Read the model definition and answer for the solid it produces. Units are mm, in the model's axes. Coordinates: 2 decimals unless noted, no trailing zeros. Order: outer loops, then holes, each group sorted by start corner. A loop starts at its lowest first (then second) coordinate and runs counter-clockwise, first axis right, second up. Notation, with made-up numbers: (-15.75, 29) -> (14.25, 29) arc R28 ccw to (14.25, 51) -> close; hole circle Ø1 at (26, -20.75). An arc over 180 degrees is marked (long way). Use CSV: the item, a comma, the result in double quotes.
```python
from build123d import *

# Parameters (mm, degrees)
BOSS_EXTRUDE1_DEPTH = 1.6
CUT_EXTRUDE2_REACH  = 117.785
SKETCH2_4_W         = 3.3
SKETCH2_4_H         = 10


with BuildPart() as part:
    # Sketch1 → Boss-Extrude1 (new, symmetric)
    with BuildSketch(Plane.XY):
        with BuildLine():
            Line((-110, 0), (110, 0))
            ThreePointArc((110, 0), (113.989001648, -3.703578255), (110.591213415, -7.956067075))
            Line((110.591213415, -7.956067075), (30, -20))
            Line((30, -20), (0, -20))
            Line((0, -20), (-30, -20))
            Line((-30, -20), (-110.591213415, -7.956067075))
            ThreePointArc((-110.591213415, -7.956067075), (-113.989001648, -3.703578255), (-110, 0))
        make_face()
    extrude(amount=BOSS_EXTRUDE1_DEPTH, both=True)

    # Sketch2<4> → Cut-Extrude2 (cut, up to next)
    with BuildSketch(Plane.XY.offset(1.6), mode=Mode.PRIVATE) as cut_extrude2_sk1:
        with Locations((0, -5)):
            Rectangle(SKETCH2_4_W, SKETCH2_4_H)
    cut_extrude2_tool1 = extrude(cut_extrude2_sk1.sketch, amount=-CUT_EXTRUDE2_REACH, mode=Mode.PRIVATE) & part.part
    add(cut_extrude2_tool1.solids().sort_by_distance((0, -5, 1.6))[0], mode=Mode.SUBTRACT)


solid = part.part
```
Item 1: Find section D-D, the plane y = -14. Give the vertices of the cut face in (x, z), then the cut area to 3 significant figures.
Return value:
outline,"(-70.15, -1.6) -> (70.15, -1.6) -> (70.15, 1.6) -> (-70.15, 1.6) -> close"
area,"449 mm^2"
Item 2: Straight lines are drawn through the part: line 1 along X through (y, z) = (-4, -1.2); line 2 along X through (y, z) = (-4.75, 1.45); line 3 along Y through (x, z) = (73, -0.35). For each, find the intervals that lie inside material, in ascending order.
Return value:
line 1,"x = -114 to -1.65, 1.65 to 114"
line 2,"x = -113.93 to -1.65, 1.65 to 113.93"
line 3,"y = -13.57 to 0"
Item 3: Find section B-B, the plane z = -0.8. Give the vertices of the cut face in (x, y).
Return value:
outline,"(-110.59, -7.96) -> (-30, -20) -> (30, -20) -> (110.59, -7.96) arc R4 ccw to (110, 0) -> (1.65, 0) -> (1.65, -10) -> (-1.65, -10) -> (-1.65, 0) -> (-110, 0) arc R4 ccw to start"
Item 4: Find section A-A, the plane y = -5.75. Give the vertices of the cut face in (x, z).
Return value:
outline,"(-113.6, -1.6) -> (-1.65, -1.6) -> (-1.65, 1.6) -> (-113.6, 1.6) -> close; (1.65, -1.6) -> (113.6, -1.6) -> (113.6, 1.6) -> (1.65, 1.6) -> close"
Item 5: Find section C-C, the plane x = 32.5. Give the vertices of the cut face in (y, z).
Return value:
outline,"(-19.63, -1.6) -> (0, -1.6) -> (0, 1.6) -> (-19.63, 1.6) -> close"
